Can you work these out from the model? Positions are in its coordinate system, mm. A direction names the side the tool comes from. Round coordinates to 2 decimals unless told otherwise and drop trailing zeros. Loops run counter-clockwise (first coordinate to the right, second up) from the corner with the lowest first, then second, coordinate; pieces in that order, holes last. Notation, with made-up numbers: (85, 57) -> (100, 57) arc R17 cw to (100, 90) -> close; hole circle Ø11 at (30.5, -24). An arc over 180 degrees is marked (long way). Answer as a JSON object with one key per item and string values.
```python
from build123d import *

# Parameters (mm, degrees)
F0_R     = 12
F1_DEPTH = 1.6
F2_R     = 11.5
F3_DEPTH = 6
F4_R     = 8
F5_DEPTH = 12
F6_R     = 2


with BuildPart() as f1:
    # F0 (on Top) → F1 (new body)
    with BuildSketch(Plane.XY):
        Circle(F0_R)
    extrude(amount=F1_DEPTH)

    # F2 (on face) → F3 (join)
    with BuildSketch(Plane.XY.offset(1.6)):
        Circle(F2_R)
    extrude(amount=F3_DEPTH)

    # F4 (on face) → F5 (join)
    with BuildSketch(Plane.XY.offset(7.6)):
        Circle(F4_R)
    extrude(amount=F5_DEPTH)

    # F6
    f6_edges = [f1.edges().sort_by_distance(p)[0] for p in [
        (-11.5, 0, 7.6),
        (-8, 0, 19.6),
    ]]
    fillet(f6_edges, radius=F6_R)


solid = f1.part
```
Q1. I want a section at D-D, the plane z = 7. Write out the boundary of the cut face in (x, y).
Determined:
{"outline": "circle Ø21.86 at (0, 0)"}
Q2. I'm going to push flat-ended pins straight in: pin 1 (1.5 mm diameter, centred on x = -4.5, y = -6, fed in from +Z); pin 2 (1 mm diameter, centred on y = -5, z = 6.5, fed in from -X); pin 3 (6 mm diameter, centred on x = -8.5, z = 6.5, fed in from -Y). Where does each tip first touch, or does it pass through?
Determined:
{"pin 1": "z = 19.45", "pin 2": "x = -10.44", "pin 3": "y = -10.04"}
Q3. I want a section at A-A, the plane y = 0. Write out the boundary of the cut face in (x, z), then the cut area to 3 significant figures.
Determined:
{"outline": "(-12, 0) -> (12, 0) -> (12, 1.6) -> (11.5, 1.6) -> (11.5, 5.6) arc R2 ccw to (9.5, 7.6) -> (8, 7.6) -> (8, 17.6) arc R2 ccw to (6, 19.6) -> (-6, 19.6) arc R2 ccw to (-8, 17.6) -> (-8, 7.6) -> (-9.5, 7.6) arc R2 ccw to (-11.5, 5.6) -> (-11.5, 1.6) -> (-12, 1.6) -> close", "area": "365 mm²"}
Q4. On a 3-axis mill with a long thin cutter (end or side, diameter ignored), from which of +Z, -Z, +X, -X, +Y, -Y can I reach the whole of each face in a straight line? I mean faces 1 (the flat face through (-4.3, -7, 7.6)), 2 (the flat face through (0, 0, 0)). Say none if no direction works.
Determined:
{"face 1": "+Z", "face 2": "-Z, +X, -X, +Y, -Y"}
Q5. I want a section at C-C, the plane z = 9. Write out the boundary of the cut face in (x, y), then the cut area to 3 significant figures.
Determined:
{"outline": "circle Ø16 at (0, 0)", "area": "201 mm²"}
Q6. If I drill on L1, parallel to Z at x = -0.75, y = 9; L2, parallel to X at y = 1.25, z = 11.25; L3, parallel to X at y = 9, z = 5, over which ranges is the centre line in solid material (lowest first)? Write a range as [from, to].
Determined:
{"L1": "[0, 7.6]", "L2": "[-7.9, 7.9]", "L3": "[-7.16, 7.16]"}
